```python
from build123d import *


with BuildPart() as f2:
    # F2: sweep along a path in F1
    with BuildLine(Plane.YZ) as f2_path:
        Line((0, 0), (0, 62.177598))
        ThreePointArc((0, 62.177598), (-3.719744, 71.157854), (-12.7, 74.877598))
        Line((-12.7, 74.877598), (-37.777253, 74.877598))
    # F0 (on Top) → F2 (sweep)
    with BuildSketch(Plane.XY):
        Polygon((-1.998463, 0.078399), (-1.067127, -1.69152), (0.931336, -1.769919), (1.998463, -0.078399), (1.067127, 1.69152), (-0.931336, 1.769919), align=None)
    sweep(path=f2_path.line)


solid = f2.part
```
The listing builds one solid part. Answer for the finished solid, in the listing's coordinates (mm). A direction names the side the tool comes from. Coordinates: 2 decimals unless noted, no trailing zeros. Write each loop counter-clockwise with the first axis right and the second up, starting at its lowest first coordinate (ties: lowest second). Pieces come first, ordered by that corner, then holes.
Q1. Which of the six approach directions +Z, -Z, +X, -X, +Y, -Y give full straight-line access (tool end or side, diameter ignored) to faces 1 (the flat face through (1.457, -0.936, 31.524)), 2 (the flat face through (0.082, -25.414, 76.608)), 3 (the flat face through (-0.08, -1.73, 31.52))?
Returned:
face 1: -Z, +X, -Y
face 2: +Z, +X, +Y, -Y
face 3: -Z, -X, -Y
Q2. Section C-C, the plane x = 0.15 is taken. Write down the section's boundary in (y, z) (1 decimal).
Returned:
outline: (-37.8, 73.1) - (-12.7, 73.1) arc R11 cw to (-1.7, 62.2) - (-1.7, 0) - (1.7, 0) - (1.7, 62.2) arc R14.4 ccw to (-12.7, 76.6) - (-37.8, 76.6) - close
Q3. Section B-B, the plane y = -25.5 is taken. Write down the section's boundary in (x, z), then the cut area to 3 significant figures.
Returned:
outline: (-2, 74.96) - (-1.07, 73.19) - (0.93, 73.11) - (2, 74.8) - (1.07, 76.57) - (-0.93, 76.65) - close
area: 10.4 mm2
Q4. Find the intervals of material crossed by line 1 along Z through (x, y) = (-0.7, -14); line 2 along Z through (x, y) = (0.7, -32); line 3 along Y through (x, z) = (-0.3, 30.5), in increasing order.
Returned:
line 1: z = 73.17 to 76.64
line 2: z = 73.12 to 76.58
line 3: y = -1.72 to 1.75
Q5. Section A-A, the plane z = 32 is taken. Write down the section's boundary in (x, y), then the cut area to 3 significant figures.
Returned:
outline: (-2, 0.08) - (-1.07, -1.69) - (0.93, -1.77) - (2, -0.08) - (1.07, 1.69) - (-0.93, 1.77) - close
area: 10.4 mm2
Q6. Given P1, Ø1, axis at y = -3.5, z = 30.5, coming from the +X side, flat-ended and moving along its own axis, determine where the tip first touches the part or whether it passes through.
Returned:
P1: passes through
